CAD build for the part. Positions are in the model's coordinates, mm. Give positions to 0.01 mm unless a question says otherwise; leave off trailing zeros. Order: outer loops, then holes, each group sorted by start corner. A loop starts at its lowest first (then second) coordinate and runs counter-clockwise, first axis right, second up.
from build123d import *

# Parameters (mm, degrees)
F0_R     = 18.9
F0_R_2   = 15.9
F1_DEPTH = 580
F5_R     = 27
F6_DEPTH = 50
F7_R     = 2.5
F8_DEPTH = 18.901


with BuildPart() as f1:
    # F0 (on Top) → F1 (new body)
    with BuildSketch(Plane.XY):
        Circle(F0_R)
        Circle(F0_R_2, mode=Mode.SUBTRACT)
    extrude(amount=F1_DEPTH)

    # F5 (on face) → F6 (cut, symmetric)
    with BuildSketch(Plane.XZ):
        with Locations((0, 580)):
            Circle(F5_R)
    extrude(amount=F6_DEPTH, both=True, mode=Mode.SUBTRACT)

    # F7 (on Right) → F8 (cut, through all)
    with BuildSketch(Plane.YZ):
        with Locations((0, 50)):
            Circle(F7_R)
    extrude(amount=F8_DEPTH, mode=Mode.SUBTRACT)


solid = f1.part
1. Saw through at B-B on y = -9. Give the cut face in (x, z), plus the area to 3 significant figures.
2. Mould opens along X. For faces 1 (the cylindrical face through (18.027, 5.677, 276.434)), 2 (the cylindrical face through (-3.45, -15.52, 275.18)), 3 (the flat face through (-4.3, 15.5, 0)) say: released by +X, released by -X, zero draft, split by the parting line, or undercut.
3. Saw through at A-A on x = 0. Give the cut face in (y, z).
4. Wall check: line 1 (X direction, y = 0, z = 217); line 2 (Y direction, x = -1.5, z = 206.5). Give the ranges that are in metal, low to high.
5. Pin check, flat tips, straight feed: P1, Ø2, axis at y = 2, z = 367.5, coming from the +X side; P2, Ø2, axis at y = -2, z = 215, coming from the -X side; P3, Ø5, axis at y = 11.5, z = 410.5, coming from the -X side; P4, Ø1, axis at x = -8, y = 14.5, coming from the -Z side. Stop position of each tip, or through.
6. Saw through at C-C on z = 502.5. Give the cut face in (x, y), plus the area to 3 significant figures.
Reported:
1. outline: (-16.62, 0) - (-13.11, 0) - (-13.11, 556.4) arc R27 cw to (-16.62, 558.72) - close; (13.11, 0) - (16.62, 0) - (16.62, 558.72) arc R27 cw to (13.11, 556.4) - close
1. area: 3,920 mm2
2. face 1: split by the parting line
2. face 2: undercut
2. face 3: zero draft
3. outline: (-18.9, 0) - (-15.9, 0) - (-15.9, 553) - (-18.9, 553) - close; (15.9, 0) - (18.9, 0) - (18.9, 553) - (15.9, 553) - close
4. line 1: x = -18.9 to -15.9, 15.9 to 18.9
4. line 2: y = -18.84 to -15.83, 15.83 to 18.84
5. P1: stops at x = 18.87
5. P2: stops at x = -18.87
5. P3: stops at x = -16.62
5. P4: stops at z = 0
6. outline: circle Ø37.8 at (0, 0); hole circle Ø31.8 at (0, 0)
6. area: 328 mm2
